Geometry check sheet. Reference: the model listing, model coordinates, mm. Face numbers are marked on the shaded views. A direction names the side the tool comes from. Coordinates: 2 decimals unless noted, no trailing zeros. Loops run counter-clockwise (first coordinate to the right, second up) from the corner with the lowest first, then second, coordinate; pieces in that order, holes last.
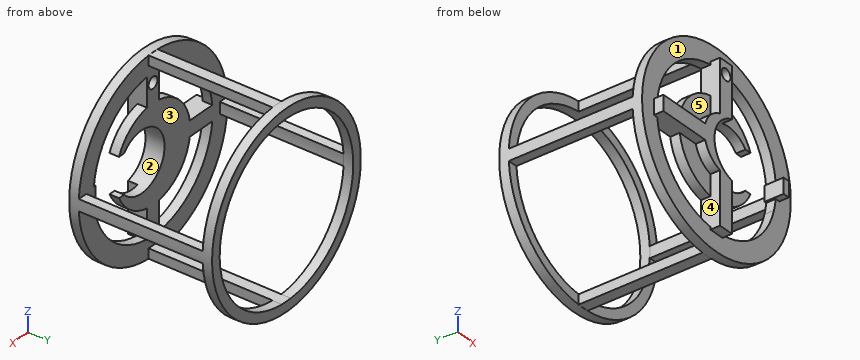
Autodesk Inventor part; units mm, degrees
ref_plane "YZ Plane" through (0, 0, 0) normal (1, 0, 0) x (0, 1, 0)
ref_plane "XZ Plane" through (0, 0, 0) normal (0, 1, 0) x (-1, 0, 0)
ref_plane "XY Plane" through (0, 0, 0) normal (0, 0, 1) x (1, 0, 0)
sketch "Szkic1" plane through (0, 0, 0) normal (0, 1, 0) x (-1, 0, 0)
  circle A0 centre (0, 0) radius 50
  dimension "d0" = 100
extrude "Wyciągnięcie proste1" add sketch "Szkic1" along normal blind 80
sketch "Szkic2" plane through (0, 80, 0) normal (0, 1, 0) x (1, 0, 0)
  circle A0 centre (0, 0) radius 45
  dimension "d3" = 90
extrude "Wyciągnięcie proste2" cut sketch "Szkic2" against normal blind 75
sketch "Szkic3" plane through (0, 5, 0) normal (0, 1, 0) x (1, 0, 0)
  point P0 (0, 0)
sketch "Szkic4" plane through (0, 5, 0) normal (0, 1, 0) x (1, 0, 0)
  circle A0 centre (0, 0) radius 7.5
  dimension "d6" = 15
extrude "Wyciągnięcie proste3" cut sketch "Szkic4" against normal blind 75
sketch "Szkic9" plane through (0, 80, 0) normal (0, 1, 0) x (1, 0, 0)
  circle A0 centre (0, 0) radius 50
  line L0 (-49.9099, 3) -> (-44.8999, 3)
  circle A1 centre (0, 0) radius 45
  line L1 (-49.9099, -3) -> (-44.8999, -3)
  line L2 (44.9005, 2.9912) -> (49.9104, 2.9912)
  line L3 (44.6345, -3) -> (49.9099, -3)
  arc A2 (-49.9099, -3) -> (49.9099, -3) centre (0, 0) ccw
  arc A3 (-40.5012, -19.6125) -> (44.6345, -3) centre (-0.1275, -0.0618) ccw
  arc A4 (49.9104, 2.9912) -> (-49.9099, 3) centre (0, 0) ccw
  arc A5 (44.9005, 2.9912) -> (-44.8999, 3) centre (-0.0001, -0.7186) ccw
  point P0 (44.9005, 2.9912)
  point P1 (44.8999, -3)
extrude "Wyciągnięcie proste4" cut sketch "Szkic9" against normal blind 75 contours L2 A1 L0 A0 | A0 L1 A1 L3 | A5 A1 | A1 L3 A3 A5 | A1 A3 L3
sketch "Szkic10" plane through (0, 80, 0) normal (0, 1, 0) x (1, 0, 0)
  circle A0 centre (0, 0) radius 50
  arc A1 (44.8999, -3) -> (44.9005, 2.9912) centre (0, 0) ccw
  circle A2 centre (0, 0) radius 45
  point P0 (44.9005, 2.9912)
extrude "Wyciągnięcie proste5" cut sketch "Szkic10" against normal blind 10
sketch "Szkic11" plane through (0, 70, 0) normal (0, 1, 0) x (1, 0, 0)
  circle A0 centre (0, 0) radius 7.5
  circle A1 centre (0, 0) radius 50
  circle A2 centre (0, 0) radius 44.8999
extrude "Wyciągnięcie proste6" add sketch "Szkic11" along normal blind 5 contours A1
sketch "Szkic12" plane through (0, 5, 0) normal (0, 1, 0) x (1, 0, 0)
  circle A0 centre (0, 0) radius 44.8999
  circle A1 centre (0, 0) radius 50
  line L0 (-3, -44.7996) -> (3, -44.7996)
  line L1 (3, -44.7996) -> (3, -49.9099)
  line L2 (3, -49.9099) -> (-3, -49.9099)
  line L3 (-3, -49.9099) -> (-3, -44.7996)
  dimension "d20" = 6
extrude "Wyciągnięcie proste7" add sketch "Szkic12" along normal blind 70 contours A0 L1 L2 L3
sketch "Szkic13" plane through (0, 5, 0) normal (0, 1, 0) x (1, 0, 0)
  arc A0 (3, -44.7996) -> (-3, -44.7996) centre (0, 0) ccw
  arc A1 (49.9104, 2.9912) -> (-49.9099, 3) centre (0, 0) ccw
  line L0 (-3, 44.7996) -> (3, 44.7996)
  line L1 (3, 44.7996) -> (3, 49.9099)
  line L2 (3, 49.9099) -> (-3, 49.9099)
  line L3 (-3, 49.9099) -> (-3, 44.7996)
  dimension "d23" = 6
extrude "Wyciągnięcie proste8" add sketch "Szkic13" along normal blind 70 contours L0 A0 | A0 L3 L2 L1
sketch "Szkic14" plane through (0, 5, 0) normal (0, 1, 0) x (1, 0, 0)
  circle A0 centre (0, 0) radius 7.5
  circle A1 centre (0, 0) radius 25
  circle A2 centre (0, 0) radius 40
  dimension "d26" = 50
  dimension "d27" = 80
extrude "Wyciągnięcie proste9" cut sketch "Szkic14" against normal blind 70 contours A2
sketch "Szkic15" plane through (0, 5, 0) normal (0, 1, 0) x (1, 0, 0)
  line L0 (-4, 41.1196) -> (4, 41.1196)
  line L1 (4, 41.1196) -> (4, -41.3332)
  line L2 (4, -41.3332) -> (-4, -41.3332)
  line L3 (-4, -41.3332) -> (-4, 41.1196)
  point P0 (0, 0)
  dimension "d30" = 8
extrude "Wyciągnięcie proste10" add sketch "Szkic15" against normal blind 10
sketch "Szkic16" plane through (0, 5, 0) normal (0, 1, 0) x (1, 0, 0)
  line L0 (-42.0523, 4) -> (42.2413, 4)
  line L1 (42.2413, 4) -> (42.2413, -4)
  line L2 (42.2413, -4) -> (-42.0523, -4)
  line L3 (-42.0523, -4) -> (-42.0523, 4)
  point P0 (0, 0)
  dimension "d33" = 8
extrude "Wyciągnięcie proste11" add sketch "Szkic16" against normal blind 10
sketch "Szkic17" plane through (0, 5, 0) normal (0, 1, 0) x (1, 0, 0)
  circle A0 centre (0, 0) radius 14.4584
extrude "Wyciągnięcie proste12" add sketch "Szkic17" against normal blind 10
sketch "Szkic18" plane through (0, 5, 0) normal (0, 1, 0) x (1, 0, 0)
  circle A0 centre (0, -35) radius 3
  point P0 (0, 0)
  dimension "d38" = 6
extrude "Wyciągnięcie proste13" cut sketch "Szkic18" against normal blind 15
sketch "Szkic22" plane through (0, 5, 0) normal (0, 1, 0) x (1, 0, 0)
  circle A0 centre (7.7599, 0) radius 15.5
  line L0 (24.6779, -4) -> (39.7995, -4)
  arc A1 (4, -39.7995) -> (39.7995, -4) centre (0, 0) ccw
  line L1 (38.713, -10.0649) -> (14.3625, -10.0649)
  line L2 (14.3625, -10.0649) -> (14.3625, 10.2037)
  line L3 (14.3625, 10.2037) -> (38.713, 10.2037)
  line L4 (38.713, 10.2037) -> (38.713, -10.0649)
  point P0 (19.4275, 10.2037)
  point P1 (19.5474, -10.0649)
  dimension "d50" = 31
extrude "Wyciągnięcie proste17" cut sketch "Szkic22" against normal blind 10 contours A0 L1 L2 L3 | A0 L3 L4 L1 | L3 L2 L1 A0
properties part number "Walec2"
1) Access from +Z, -Z, +X, -X, +Y, -Y to the whole of each face (thin tool, end or side, straight path). Record for the marked faces 3, 4 and 5.
Data:
face 3: none
face 4: -Y
face 5: +Z, -X, -Y
2) Section check B-B on y = 22.5. Record the cut outline in (x, z).
Data:
outline: (-49.91, -3) - (-44.9, -3) arc R45 cw to (-44.9, 3) - (-49.91, 3) arc R50 ccw to start; (-3, -49.91) - (3, -49.91) - (3, -44.8) - (-3, -44.8) - close; (-3, 44.8) arc R44.9 cw to (3, 44.8) - (3, 49.91) - (-3, 49.91) - close; (44.9, -2.99) - (49.91, -2.99) arc R50 ccw to (49.91, 3) - (44.9, 3) arc R45 cw to start
3) Mould release check, pull along Z, two halves, no side actions. Record for the marked faces 1 and 2: +Z half, -Z half, draft (parallel to the pull), parting line (faces both ways), or undercut.
Data:
face 1: draft
face 2: undercut
4) Depth check by flat-ended pin: pin 1 (6 mm diameter, centred on x = -16, z = -19, fed in from -Y); pin 2 (2.5 mm diameter, centred on y = 48, z = -48, fed in from -X); pin 3 (2.5 mm diameter, centred on x = -47, y = 29, fed in from -Z). Enter the tip coordinate at first touch or a pass-through.
Data:
pin 1: stops at y = 0
pin 2: stops at x = -3
pin 3: stops at z = -3
5) Material ranges on probe 1 along X at (y, z) = (-2, 35); probe 2 along Z at (x, y) = (0, 2); probe 3 along X at (y, z) = (21, 0), recorded low to high.
Data:
probe 1: x = -4 to -3, 3 to 4
probe 2: z = -50 to -13.42, 13.42 to 32, 38 to 50
probe 3: x = -50 to -45, 45 to 50
6) Section check A-A on z = 35. Record the cut outline in (x, y), and give its area (3 significant figures).
Data:
outline: (-35.71, 0) - (-19.36, 0) - (-19.36, 5) - (-35.71, 5) - close; (-35.71, 70) - (-28.12, 70) - (-28.12, 75) - (-35.71, 75) - close; (-4, -5) - (-3, -5) - (-3, 5) - (-4, 5) - close; (3, -5) - (4, -5) - (4, 5) - (3, 5) - close; (19.36, 0) - (35.71, 0) - (35.71, 5) - (19.36, 5) - close; (28.12, 70) - (35.71, 70) - (35.71, 75) - (28.12, 75) - close
area: 259 mm2
